The figure shows three views and two pictorial views of one solid part (mm, origin at its lowest corner). Answer the questions. A direction names the side the tool comes from. Round coordinates to 2 decimals unless told otherwise and drop trailing zeros. Loops run counter-clockwise (first coordinate to the right, second up) from the corner with the lowest first, then second, coordinate; pieces in that order, holes last. Notation, with made-up numbers: (1, -31) -> (8, -31) arc R31 ccw to (8, -2) -> close; hole circle Ø6 at (87, 22.5). An arc over 180 degrees is marked (long way). Write each question's results on one line, items separated by ' | '. Start each with the question number.
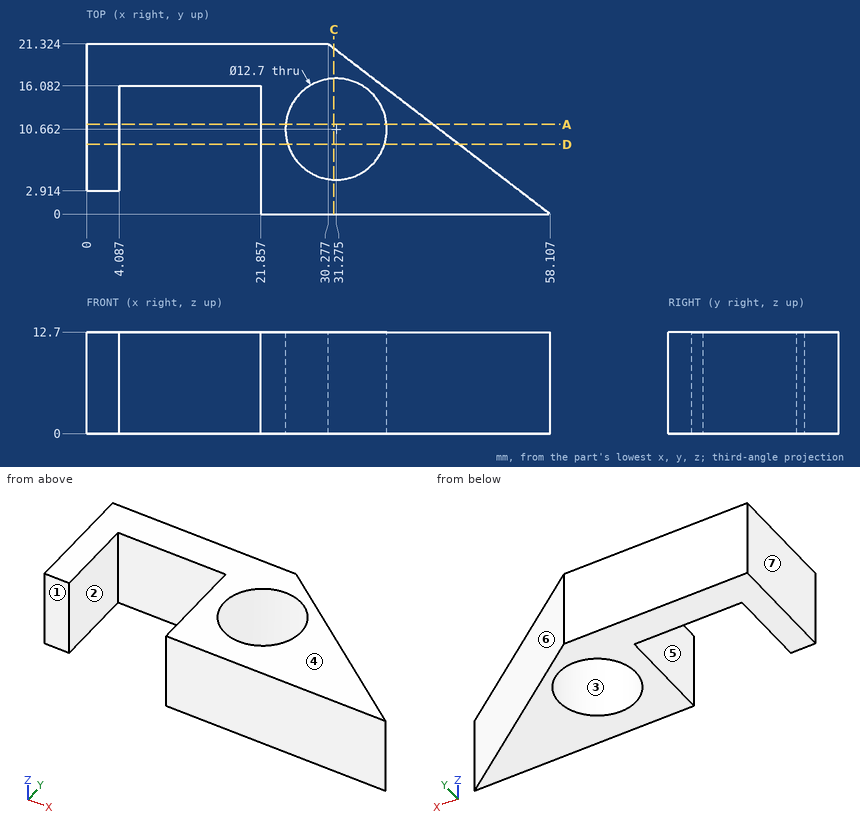
Item 1: The part is cut by section C-C, the plane x = 31. Give the vertices of the cut face in (y, z) (1 decimal), plus the area to 3 significant figures.
Item 2: The part is cut by section A-A, the plane y = 11.25. Give the vertices of the cut face in (x, z) (1 decimal), plus the area to 3 significant figures.
Item 3: The part is cut by section D-D, the plane y = 8.75. Give the vertices of the cut face in (x, z).
Item 4: Each of these flat-tipped pins is pushed along its axis until it touches: pin 1 Ø6 at (x, z) = (18.5, 10.5) entering from -Y; pin 2 Ø3 at (x, y) = (36.5, 19) entering from -Z; pin 3 Ø2 at (y, z) = (4, 1.5) entering from +X; pin 4 Ø2 at (x, z) = (1.5, 8.5) entering from -Y. Where does it stop, or does it pass through?
Item 5: Determine the mould class of the marked faces 4, 5, 6 and 7 for opening direction X: +X half, -X half, draft (parallel to the pull), parting line (faces both ways), or undercut.
Item 6: Straight lines are drawn through the part: L1, parallel to X at y = 15.5, z = 5 (1 decimal); L2, parallel to X at y = 13.5, z = 6.5 (1 decimal); L3, parallel to Y at x = 30, z = 7.75. For each, find the intervals that lie inside material, in ascending order. Write a range as [from, to].
Item 7: For the marked faces 1, 2 and 3, determine the directions among +Z, -Z, +X, -X, +Y, -Y from which every point of the face is accessible in a straight line to the end or side of a thin tool.
Report:
1) outline: (0, 0) -> (4.3, 0) -> (4.3, 12.7) -> (0, 12.7) -> close; (17, 0) -> (20.8, 0) -> (20.8, 12.7) -> (17, 12.7) -> close | area: 103 mm2
2) outline: (0, 0) -> (4.1, 0) -> (4.1, 12.7) -> (0, 12.7) -> close; (21.9, 0) -> (25, 0) -> (25, 12.7) -> (21.9, 12.7) -> close; (37.6, 0) -> (43.4, 0) -> (43.4, 12.7) -> (37.6, 12.7) -> close | area: 165 mm2
3) outline: (0, 0) -> (4.09, 0) -> (4.09, 12.7) -> (0, 12.7) -> close; (21.86, 0) -> (25.22, 0) -> (25.22, 12.7) -> (21.86, 12.7) -> close; (37.33, 0) -> (46.69, 0) -> (46.69, 12.7) -> (37.33, 12.7) -> close
4) pin 1: stops at y = 16.08 | pin 2: passes through | pin 3: stops at x = 54.19 | pin 4: stops at y = 2.91
5) face 4: draft | face 5: undercut | face 6: +X half | face 7: -X half
6) L1: x = [0, 4.1], [21.9, 27.2], [35.4, 37.9] | L2: x = [0, 4.1], [21.9, 25.6], [37, 40.5] | L3: y = [0, 4.44], [16.88, 21.32]
7) face 1: +Z, -Z, -X, -Y | face 2: +Z, -Z, -Y | face 3: +Z, -Z
